Verification items for the finished model (mm, model axes). Coordinates: 2 decimals unless noted, no trailing zeros. Write each loop counter-clockwise with the first axis right and the second up, starting at its lowest first coordinate (ties: lowest second). Pieces come first, ordered by that corner, then holes. Notation, with made-up numbers: M 22,-28.5 L 61,-28.5 A26 cw 61,2.5 Z; hole C -12,69 d1. An arc over 180 degrees is marked long. Answer in a Markdown table with one row per item.
from build123d import *

# Parameters (mm, degrees)
SKETCH1_W                      = 38.1
SKETCH1_H                      = 88.9
BOSS_EXTRUDE1_DEPTH            = 431.8
F_5_16_0_3125_DIAMETER_HOLE1_D = 7.9375


with BuildPart() as part:
    # Sketch1 → Boss-Extrude1 (new body)
    with BuildSketch(Plane.XY):
        Rectangle(SKETCH1_W, SKETCH1_H)
    extrude(amount=BOSS_EXTRUDE1_DEPTH)

    # 5/16 (0.3125) Diameter Hole1 (through all)
    with Locations(Plane(origin=(19.05, 0, 0), x_dir=(0, 0, -1), z_dir=(1, 0, 0))):
        with Locations((-393.7, 0), (-38.1, 0)):
            Hole(F_5_16_0_3125_DIAMETER_HOLE1_D / 2)


solid = part.part
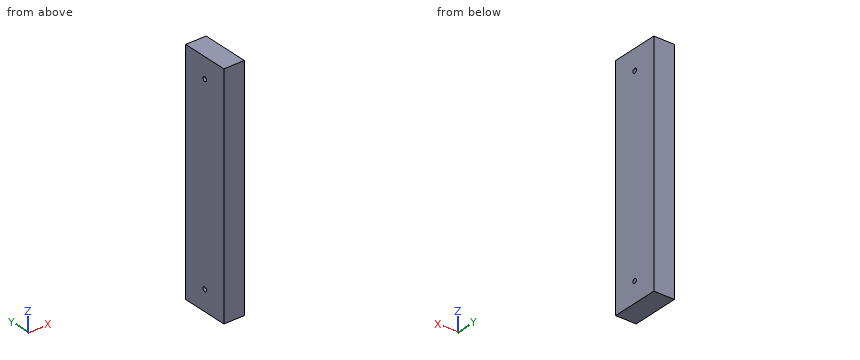
1) Sectioned sample at A-A (z = 38.1). Record the cut outline in (x, y), then the cut area to 3 significant figures.
Response values:
| item | result |
|---|---|
| outline | M -19.05,-44.45 L 19.05,-44.45 L 19.05,-3.97 L -19.05,-3.97 Z; M -19.05,3.97 L 19.05,3.97 L 19.05,44.45 L -19.05,44.45 Z |
| area | 3,080 mm² |
2) Thickness scan on L1, parallel to Y at x = 11, z = 38; L2, parallel to Y at x = 9, z = 393. Record the ranges inside material, lowest first. Write a range as [from, to].
Response values:
| item | result |
|---|---|
| L1 | y = [-44.45, -3.97], [3.97, 44.45] |
| L2 | y = [-44.45, -3.91], [3.91, 44.45] |
3) Depth check by flat-ended pin: pin 1 (6.5 mm diameter, centred on y = 0, z = 393.7, fed in from -X). Enter the tip coordinate at first touch or a pass-through.
Response values:
| item | result |
|---|---|
| pin 1 | passes through |
4) Sectioned sample at B-B (y = 0). Record the cut outline in (x, z), then the cut area to 3 significant figures.
Response values:
| item | result |
|---|---|
| outline | M -19.05,0 L 19.05,0 L 19.05,34.13 L -19.05,34.13 Z; M -19.05,42.07 L 19.05,42.07 L 19.05,389.73 L -19.05,389.73 Z; M -19.05,397.67 L 19.05,397.67 L 19.05,431.8 L -19.05,431.8 Z |
| area | 15,800 mm² |
